from build123d import *

# Parameters (mm, degrees)
IZIM1_R                     = 6
Y_KSEKLIK_EKSTR_ZYON1_DEPTH = 150
IZIM2_W                     = 35
IZIM2_H                     = 18.169429668
Y_KSEKLIK_EKSTR_ZYON2_DEPTH = 105
RADYUS1_R                   = 8
M3_BO_LUKLU_DELIK1_D        = 3.4
KES_EKSTR_ZYON1_START       = -105
IZIM8_R                     = 6
KES_EKSTR_ZYON1_DEPTH       = 105
IZIM9_R                     = 6.319148562
KES_EKSTR_ZYON2_DEPTH       = 10


with BuildPart() as part:
    # Çizim1 → Yükseklik-Ekstrüzyon1 (new body)
    with BuildSketch(Plane.XY):
        with BuildLine():
            Line((0, -23.530781845), (8.315682398, -3.44229956))
            ThreePointArc((8.315682398, -3.44229956), (0, 9), (-8.315682398, -3.44229956))
            Line((-8.315682398, -3.44229956), (0, -23.530781845))
        make_face()
        Circle(IZIM1_R, mode=Mode.SUBTRACT)
    extrude(amount=Y_KSEKLIK_EKSTR_ZYON1_DEPTH)

    # Çizim2 → Yükseklik-Ekstrüzyon2 (add)
    with BuildSketch(Plane.XY):
        Rectangle(IZIM2_W, IZIM2_H)
    extrude(amount=-Y_KSEKLIK_EKSTR_ZYON2_DEPTH)

    # Radyus1
    radyus1_edges = [part.edges().sort_by_distance(p)[0] for p in [
        (17.5, 0, 0),
        (-17.5, 0, 0),
    ]]
    fillet(radyus1_edges, radius=RADYUS1_R)

    # M3 Boşluklu Delik1 (through all)
    with Locations(Plane(origin=(0, 9.084714834, 0), x_dir=(1, 0, 0), z_dir=(0, 1, 0))):
        with Locations((-12.5, 80), (12.5, 80), (0, 100)):
            Hole(M3_BO_LUKLU_DELIK1_D / 2)

    # Çizim8 → Kes-Ekstrüzyon1 (cut)
    with BuildSketch(Plane.XY.offset(KES_EKSTR_ZYON1_START)):
        Circle(IZIM8_R)
    extrude(amount=KES_EKSTR_ZYON1_DEPTH, mode=Mode.SUBTRACT)

    # Çizim9 → Kes-Ekstrüzyon2 (cut)
    with BuildSketch(Plane.XZ.offset(9.084714834)):
        with Locations(Location((0, -11.539481772, 0), (0, 0, 270))):
            Circle(IZIM9_R)
    extrude(amount=-KES_EKSTR_ZYON2_DEPTH, mode=Mode.SUBTRACT)


solid = part.part
Source: CAD feature listing. Evaluate the final solid. Frame: model axes, mm. A direction names the side the tool comes from. Give positions to 0.01 mm unless a question says otherwise; leave off trailing zeros. Write each loop counter-clockwise with the first axis right and the second up, starting at its lowest first coordinate (ties: lowest second). Pieces come first, ordered by that corner, then holes. Notation, with made-up numbers: (12.25, -33) -> (16.25, -33) arc R27 cw to (16.25, 6) -> close; hole circle Ø7 at (46.25, 56.5). An arc over 180 degrees is marked (long way). Write item = value, one per line.
Q1. Line query: line 1 (X direction, y = 0, z = 39); line 2 (Y direction, x = 0, z = 91.5); line 3 (X direction, y = -3.75, z = -80). Output: solid intervals per line, ascending. Write a range as from..to.
Here are the results:
line_1 = -9..-6, 6..9
line_2 = -23.53..-6, 6..9
line_3 = -17.5..-14.2, -10.8..-4.68, 4.68..10.8, 14.2..17.5
Q2. First-contact query: pin 1 (3 mm diameter, centred on x = 0, z = -100, fed in from -Y); pin 2 (5.5 mm diameter, centred on x = 0, z = -100, fed in from -Y); pin 3 (3 mm diameter, centred on y = -12.5, z = 116.5, fed in from -X); pin 4 (8 mm diameter, centred on x = 9, z = 44, fed in from +Y). Flat tips, straight axial feed; report the tip coordinate or a pass-through.
Here are the results:
pin_1 = through
pin_2 = -9.08
pin_3 = -5.19
pin_4 = 7.48
Q3. Cut plane A-A on y = 3. Return loops of the section in (x, z), then the cut area to 3 significant figures.
Here are the results:
outline = (-17.5, -105) -> (-5.2, -105) -> (-5.2, 150) -> (-8.49, 150) -> (-8.49, 0) -> (-9.5, 0) arc R8 ccw to (-17.5, -8) -> close; (5.2, -105) -> (17.5, -105) -> (17.5, -8) arc R8 ccw to (9.5, 0) -> (8.49, 0) -> (8.49, 150) -> (5.2, 150) -> close; hole circle Ø3.4 at (-12.5, -80); hole circle Ø3.4 at (12.5, -80)
area = 3,520 mm²
Q4. Cut plane C-C on z = 117.5. Return loops of the section in (x, y).
Here are the results:
outline = (-8.32, -3.44) -> (0, -23.53) -> (8.32, -3.44) arc R9 ccw (long way) to start; hole circle Ø12 at (0, 0)
Q5. Reachability of faces 5 (the face through (-15.219, 0.127, -2.406)), 6 (the face through (4.1, -13.63, 73.95)), 7 (the face through (-0.2, 6.2, -105)), 8 (the face through (0, -15, 0)), 9 (the face through (0, 9, 74)) from +Z, -Z, +X, -X, +Y, -Y: full face, straight path, thin tool, end or side. Return the list, or none.
Here are the results:
face_5 = +Z, -X, +Y, -Y
face_6 = +Z, +X, -Y
face_7 = -Z, +X, -X, +Y, -Y
face_8 = -Z, +X, -X, -Y
face_9 = +Z
Q6. Mould query, pull axis X, two halves, no side actions, for faces 1 (the face through (-4.216, -13.346, 73.95)), 2 (the face through (-3.845, -5.266, -6.525)), 3 (the face through (0, -9.085, -52)), 4 (the face through (15.094, 0.127, -2.281)). Classes: +X half, -X half, draft (parallel to the pull), parting line (faces both ways), or undercut.
Here are the results:
face_1 = -X half
face_2 = undercut
face_3 = draft
face_4 = +X half
Q7. Cut plane B-B on z = -51. Return loops of the section in (x, y), then the cut area to 3 significant figures.
Here are the results:
outline = (-17.5, -9.08) -> (17.5, -9.08) -> (17.5, 9.08) -> (-17.5, 9.08) -> close; hole circle Ø12 at (0, 0)
area = 523 mm²
